Check sheet for the modelled part. Datum: model origin and axes. Units: mm. A direction names the side the tool comes from. Coordinates: 2 decimals unless noted, no trailing zeros. Loops run counter-clockwise (first coordinate to the right, second up) from the corner with the lowest first, then second, coordinate; pieces in that order, holes last. Notation, with made-up numbers: M -28.75,38.25 L 18.25,38.25 A31 cw 18.25,75.25 Z; hole C 71,57 d2. An arc over 180 degrees is marked long. Return JSON: item names as keys, results as strings.
from build123d import *

# Parameters (mm, degrees)
SKETCH2_R           = 60
BOSS_EXTRUDE1_DEPTH = 100
SKETCH3_R           = 30
CUT_EXTRUDE1_DEPTH  = 132.148770486
SKETCH4_W           = 18
SKETCH4_H           = 11
CUT_EXTRUDE2_DEPTH  = 132.148770486


with BuildPart() as part:
    # Sketch2 → Boss-Extrude1 (new body)
    with BuildSketch(Plane(origin=(0, 0, 0), x_dir=(1, 0, 0), z_dir=(0, 1, 0))):
        with Locations(Location((0, 0, 0), (0, 0, 270))):
            Circle(SKETCH2_R)
    extrude(amount=BOSS_EXTRUDE1_DEPTH)

    # Sketch3 → Cut-Extrude1 (cut, through all)
    with BuildSketch(Plane(origin=(0, 100, 0), x_dir=(1, 0, 0), z_dir=(0, 1, 0))):
        with Locations(Location((0, 0, 0), (0, 0, 270))):
            Circle(SKETCH3_R)
    extrude(amount=-CUT_EXTRUDE1_DEPTH, mode=Mode.SUBTRACT)

    # Sketch4 → Cut-Extrude2 (cut, through all)
    with BuildSketch(Plane(origin=(0, 100, 0), x_dir=(1, 0, 0), z_dir=(0, 1, 0))):
        with Locations((0, 28.9)):
            Rectangle(SKETCH4_W, SKETCH4_H)
    extrude(amount=-CUT_EXTRUDE2_DEPTH, mode=Mode.SUBTRACT)


solid = part.part
1) Section check C-C on y = 53.5. Record the cut outline in (x, z).
Answers:
{"outline": "C 0,0 d120; hole M -9,-34.4 L 9,-34.4 L 9,-28.62 A30 ccw long -9,-28.62 Z"}
2) Section check D-D on x = 38. Record the cut outline in (y, z).
Answers:
{"outline": "M 0,-46.43 L 100,-46.43 L 100,46.43 L 0,46.43 Z"}
3) Set-up check for faces 4 (the face through (28, 0, 12)), 5 (the face through (-9, 51, -31)): record each of +Z, -Z, +X, -X, +Y, -Y from which the full face is reachable in a straight line by a thin tool's end or side.
Answers:
{"face 4": "+Z, -Z, +X, -X, -Y", "face 5": "+Y, -Y"}
4) Section check A-A on x = 0. Record the cut outline in (y, z).
Answers:
{"outline": "M 0,-60 L 100,-60 L 100,-34.4 L 0,-34.4 Z; M 0,30 L 100,30 L 100,60 L 0,60 Z"}
5) Section check B-B on z = 0. Record the cut outline in (x, y), then the cut area to 3 significant figures.
Answers:
{"outline": "M -60,0 L -30,0 L -30,100 L -60,100 Z; M 30,0 L 60,0 L 60,100 L 30,100 Z", "area": "6,000 mm²"}
6) Scan lines: line 1 along X through (y, z) = (53, 0); line 2 along X through (y, z) = (17, 21); line 3 along Z through (x, y) = (-2.5, 53). Record each from-to range of solid material in increasing order. Write a range as [from, to].
Answers:
{"line 1": "[-60, -30], [30, 60]", "line 2": "[-56.2, -21.42], [21.42, 56.2]", "line 3": "[-59.95, -34.4], [29.9, 59.95]"}
7) Go/stop test with flat-tipped pins: pin 1 Ø4.5 at (y, z) = (47, -32) entering from -X; pin 2 Ø12 at (x, y) = (35, 71.5) entering from +Z; pin 3 Ø4 at (y, z) = (84, -12) entering from -X. Record where each tip stops, or that it passes through.
Answers:
{"pin 1": "x = -52.11", "pin 2": "z = 52.53", "pin 3": "x = -59.16"}
8) Draft check along X on faces 1 (the face through (2.64, 49.3, -59.94)), 2 (the face through (9, 51, -31)), 3 (the face through (28, 100, 12)). Enter one of: +X half, -X half, draft (parallel to the pull), parting line (faces both ways), or undercut.
Answers:
{"face 1": "parting line", "face 2": "undercut", "face 3": "draft"}
